Part print with two shaded views. Sizes in mm from the minimum x, y, z corner. Round coordinates to 2 decimals unless told otherwise and drop trailing zeros. Order: outer loops, then holes, each group sorted by start corner. A loop starts at its lowest first (then second) coordinate and runs counter-clockwise, first axis right, second up. Notation, with made-up numbers: M 64.5,-33 L 123.5,-33 A17 cw 123.5,-25 Z; hole C 84,22 d11. An arc over 180 degrees is marked long. One line per question, with ' | ' between items. Start each with the question number.
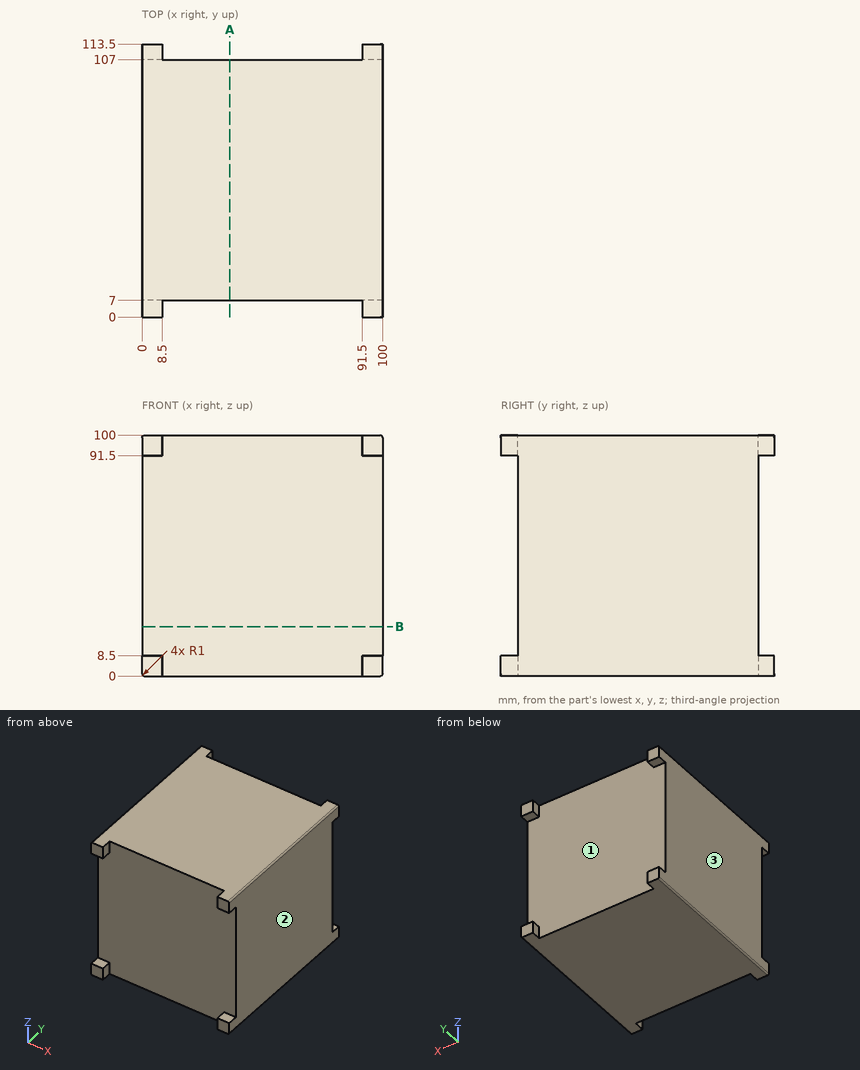
Item 1: Two-plate mould, pull along X, no slides. Class the marked faces 1, 2 and 3: +X half, -X half, draft (parallel to the pull), parting line (faces both ways), or undercut.
Item 2: Flat gauge pins, fed straight in: pin 1 (2 mm diameter, centred on x = 56.5, z = 60, fed in from +Y); pin 2 (12 mm diameter, centred on x = 39, z = 74.5, fed in from -Y). Where does each tip first touch, or does it go through?
Item 3: Cut at A-A on x = 36.5. Write the cut outline in (y, z), then the cut area to 3 significant figures.
Item 4: Wall check: line 1 along Y through (x, z) = (46, 52.5). Give the ranges that are in metal, low to high. Write a range as [from, to].
Item 5: Cut at B-B on z = 20.5. Write the cut outline in (x, y).
Results found:
1) face 1: undercut | face 2: +X half | face 3: -X half
2) pin 1: stops at y = 107 | pin 2: stops at y = 7
3) outline: M 7,0 L 107,0 L 107,100 L 7,100 Z | area: 10,000 mm^2
4) line 1: y = [7, 107]
5) outline: M 0,7 L 100,7 L 100,107 L 0,107 Z
